Here's the drawing with two shaded views (mm, measured from the low corner). I have some questions. A direction names the side the tool comes from. Coordinates: 2 decimals unless noted, no trailing zeros. Loops run counter-clockwise (first coordinate to the right, second up) from the corner with the lowest first, then second, coordinate; pieces in that order, holes last. Notation, with made-up numbers: M 89.25,29 L 144.25,29 A10 cw 144.25,47 Z; hole C -6.75,66.25 d3. An arc over 180 degrees is marked long. Return JSON: item names as keys, results as strings. Group by question number.
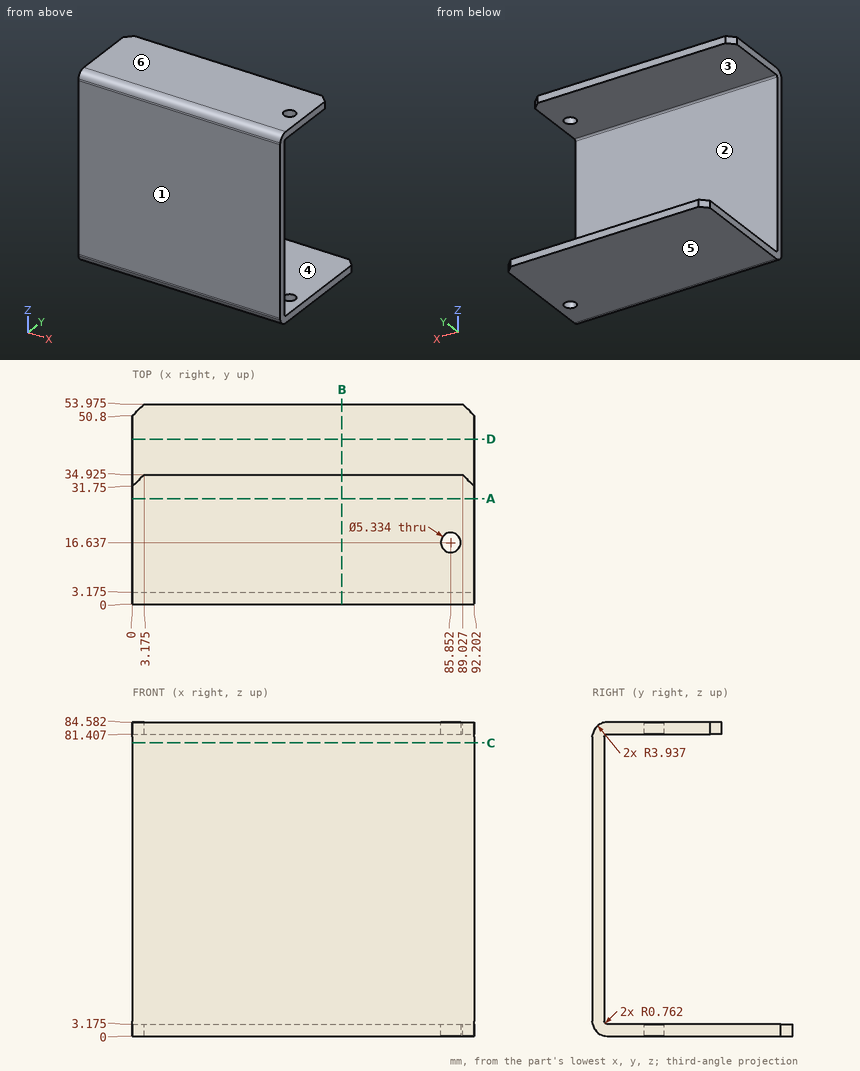
(1) We'd pull the mould along Z, two halves only. Please class the marked faces 3, 4, 5 and 6: +Z half, -Z half, draft (parallel to the pull), parting line (faces both ways), or undercut.
(2) For the marked faces 1 and 2, which set-ups out of +Z, -Z, +X, -X, +Y, -Y let a thin tool reach every point of the face, with its end or its side?
(3) Imagine slicing it at A-A, the plane y = 28.5. Write out the boundary of the cut face in (x, z) (3 decimals).
(4) Imagine slicing it at C-C, the plane z = 79. Write out the boundary of the cut face in (x, y) (3 decimals).
(5) Imagine slicing it at B-B, the plane x = 56.5. Write out the boundary of the cut face in (y, z) (3 decimals), then the cut area to 3 significant figures.
(6) Will these pins go through, and if not, where does the flat tip stop? P1, Ø6, axis at x = 85.852, y = 16.637, coming from the -Z side; P2, Ø6, axis at x = 64.5, z = 69.5, coming from the +Y side (3 decimals); P3, Ø3.5, axis at x = 30.5, z = 82.5, coming from the +Y side (3 decimals).
(7) If I drill on L1, parallel to Z at x = 45.5, y = 8.5 (3 decimals); L2, parallel to Y at x = 88, z = 41 (3 decimals), over which ranges is the centre line in solid material (lowest first)? Write a range as [from, to].
Checks:
{
 "1": {"face 3": "undercut", "face 4": "undercut", "face 5": "-Z half", "face 6": "+Z half"},
 "2": {"face 1": "+Z, -Z, +X, -X, -Y", "face 2": "+X, -X, +Y"},
 "3": {"outline": "M 0,0 L 92.202,0 L 92.202,3.175 L 0,3.175 Z; M 0,81.407 L 92.202,81.407 L 92.202,84.582 L 0,84.582 Z"},
 "4": {"outline": "M 0,0 L 92.202,0 L 92.202,3.175 L 0,3.175 Z"},
 "5": {"outline": "M 0,3.937 A3.937 ccw 3.937,0 L 53.975,0 L 53.975,3.175 L 3.937,3.175 A0.762 cw 3.175,3.937 L 3.175,80.645 A0.762 cw 3.937,81.407 L 34.925,81.407 L 34.925,84.582 L 3.937,84.582 A3.937 ccw 0,80.645 Z", "area": "524 mm²"},
 "6": {"P1": "z = 0", "P2": "y = 3.175", "P3": "y = 34.925"},
 "7": {"L1": "[0, 3.175], [81.407, 84.582]", "L2": "[0, 3.175]"}
}
